```python
from build123d import *

# Parameters (mm, degrees)
BOSS_EXTRUDE1_DEPTH     = 12.7
SKETCH2_R               = 5.08
BOSS_EXTRUDE2_DEPTH     = 25.4
CUT_EXTRUDE1_DEPTH      = 6.858
CUT_EXTRUDE1_DEPTH_BACK = 12.954
SKETCH3_R               = 3.81


with BuildPart() as part:
    # Sketch1 → Boss-Extrude1 (new body)
    with BuildSketch(Plane.XY):
        with BuildLine():
            Line((-5.436566547, 31.20219701), (37.743433453, 28.02719701))
            ThreePointArc((37.743433453, 28.02719701), (44.093433453, 21.67719701), (37.743433453, 15.32719701))
            Line((37.743433453, 15.32719701), (-5.436566547, 12.15219701))
            add(Edge.make_bspline(
                [(-5.436566547, 12.15219701), (-10.516566547, 21.67719701), (-5.436566547, 31.20219701)],
                knots=[0, 0, 0, 1, 1, 1], degree=2))
        make_face()
    extrude(amount=BOSS_EXTRUDE1_DEPTH)

    # Sketch2 → Boss-Extrude2 (add)
    with BuildSketch(Plane.XY):
        with Locations((37.743433453, 21.67719701)):
            Circle(SKETCH2_R)
    extrude(amount=BOSS_EXTRUDE2_DEPTH)

    # Sketch3 → Cut-Extrude1 (cut, two sides: drawn at the far end of the back side and taken through both)
    with BuildSketch(Plane.XY.offset(12.7).offset(-CUT_EXTRUDE1_DEPTH_BACK)):
        with Locations((16.915433453, 21.67719701)):
            Circle(SKETCH3_R)
    extrude(amount=CUT_EXTRUDE1_DEPTH + CUT_EXTRUDE1_DEPTH_BACK, mode=Mode.SUBTRACT)


solid = part.part
```
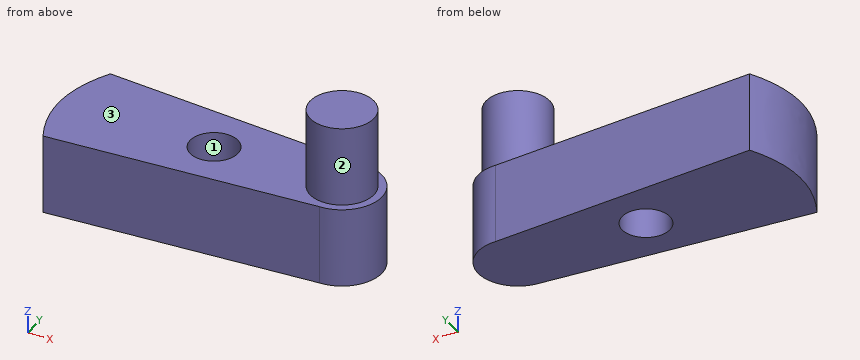
The listing builds one solid part. Answer for the finished solid, in the listing's coordinates (mm). Face numbers are marked on the shaded views. Give positions to 0.01 mm unless a question says otherwise; leave off trailing zeros. Order: outer loops, then holes, each group sorted by start corner. A loop starts at its lowest first (then second) coordinate and runs counter-clockwise, first axis right, second up. Notation, with made-up numbers: (-30.75, -24) - (-16.75, -24) arc R22 cw to (-16.75, -1) - close; hole circle Ø1 at (26.25, -1). An arc over 180 degrees is marked (long way). Use one line per item in the form item = value. Start each with the question number.
(1) Consider line 1 (Z direction, x = -3, y = 28.5); line 2 (Y direction, x = 17, z = 2.25); line 3 (X direction, y = 20.5, z = 9.5). Determine where each line is inside the solid, lowest interval first. Write a range as from..to.
(2) A cutting plane is placed at C-C, the plane z = 17.75. Write down the section's boundary in (x, y).
(3) A cutting plane is placed at D-D, the plane x = 5.5. Write down the section's boundary in (y, z), then the cut area to 3 significant figures.
(4) Flat-ended cylindrical pins translate along their axes: pin 1 Ø6 at (x, y) = (12.5, 22) entering from +Z; pin 2 Ø12 at (x, z) = (22, 13.5) entering from -Y; pin 3 Ø12 at (x, z) = (6, 7.5) entering from -Y. Find the tip coordinate at first contact, or state that the pin passes through.
(5) A cutting plane is placed at A-A, the plane x = 18. Write down the section's boundary in (y, z).
(6) A cutting plane is placed at B-B, the plane x = 12. Write down the section's boundary in (y, z), then the cut area to 3 significant figures.
(7) The mould has two halves that part along X. Classify the marked faces 1, 2 and 3: released by +X, released by -X, zero draft, split by the parting line, or undercut.
Ans:
q1.line_1 = 0..12.7
q1.line_2 = 13.8..17.87, 25.49..29.55
q1.line_3 = -7.94..13.29, 20.54..43.98
q2.outline = circle Ø10.16 at (37.74, 21.68)
q3.outline = (12.96, 0) - (30.4, 0) - (30.4, 12.7) - (12.96, 12.7) - close
q3.area = 222 mm^2
q4.pin_1 = 12.7
q4.pin_2 = 13.73
q4.pin_3 = 12.55
q5.outline = (13.88, 0) - (18.02, 0) - (18.02, 12.7) - (13.88, 12.7) - close; (25.33, 0) - (29.48, 0) - (29.48, 12.7) - (25.33, 12.7) - close
q6.outline = (13.43, 0) - (29.92, 0) - (29.92, 12.7) - (13.43, 12.7) - close
q6.area = 209 mm^2
q7.face_1 = undercut
q7.face_2 = split by the parting line
q7.face_3 = zero draft
